Source: CAD feature listing. Evaluate the final solid. Frame: model axes, mm. Face numbers are marked on the shaded views. Give positions to 0.01 mm unless a question says otherwise; leave off trailing zeros. Loops run counter-clockwise (first coordinate to the right, second up) from the corner with the lowest first, then second, coordinate; pieces in that order, holes last.
from build123d import *

# Parameters (mm, degrees)
SALIENTE_EXTRUIR1_DEPTH = 140
SALIENTE_EXTRUIR2_START = 13.3
SALIENTE_EXTRUIR2_DEPTH = 8
SALIENTE_EXTRUIR3_START = 119
SALIENTE_EXTRUIR3_DEPTH = 8


with BuildPart() as part:
    # Croquis1 → Saliente-Extruir1 (new body)
    with BuildSketch(Plane(origin=(0, 0, 0), x_dir=(0, 0, -1), z_dir=(1, 0, 0))):
        Polygon((-70.251247354, -24.917082451), (71.151247354, 22.217082451), (70.251247354, 24.917082451), (-71.151247354, -22.217082451), align=None)
    extrude(amount=SALIENTE_EXTRUIR1_DEPTH)

    # Croquis1_3 → Saliente-Extruir2 (add)
    with BuildSketch(Plane(origin=(0, 0, 0), x_dir=(0, 0, -1), z_dir=(1, 0, 0)).offset(SALIENTE_EXTRUIR2_START)):
        Polygon((57.348752646, 17.616250882), (-39.651247354, -14.717082451), (-39.651247354, -22.717082451), (57.348752646, 9.616250882), align=None)
    extrude(amount=SALIENTE_EXTRUIR2_DEPTH)

    # Croquis1_4 → Saliente-Extruir3 (add)
    with BuildSketch(Plane(origin=(0, 0, 0), x_dir=(0, 0, -1), z_dir=(1, 0, 0)).offset(SALIENTE_EXTRUIR3_START)):
        Polygon((57.348752646, 17.616250882), (-39.651247354, -14.717082451), (-39.651247354, -22.717082451), (57.348752646, 9.616250882), align=None)
    extrude(amount=SALIENTE_EXTRUIR3_DEPTH)


solid = part.part
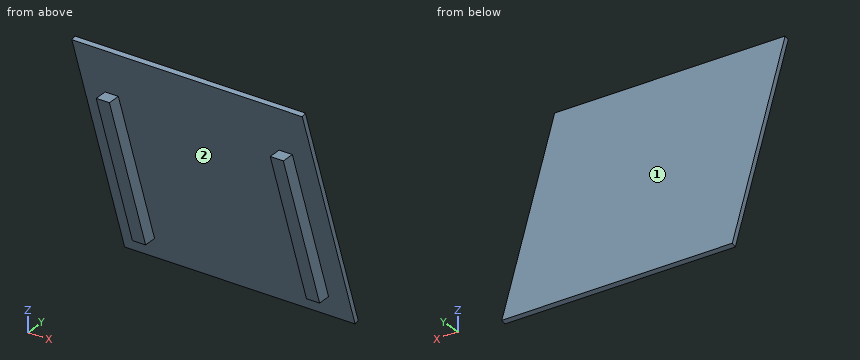
1) Contact query for flat-ended pins moving along their axis: P1, Ø20, axis at y = -7, z = -15.5, coming from the -X side; P2, Ø9, axis at x = 122.5, y = -20, coming from the +Z side; P3, Ø4, axis at x = 16.5, y = 12, coming from the -Z side; P4, Ø20, axis at y = -12, z = -20.5, coming from the +X side. Output: stop coordinate, or through.
Checks:
P1: stops at x = 13.3
P2: stops at z = 71.15
P3: stops at z = -57.35
P4: stops at x = 127
2) Pull-direction query (X, two-part tool) for the marked faces 1 and 2; classes: released by +X, released by -X, zero draft, split by the parting line, or undercut.
Checks:
face 1: zero draft
face 2: undercut
3) Cut plane D-D (x = 38.5). Return loops of the section in (y, z).
Checks:
outline: (-24.92, 70.25) - (22.22, -71.15) - (24.92, -70.25) - (-22.22, 71.15) - close
4) Ray query, probe 1 along X at (y, z) = (-17, 28); probe 2 along Y at (x, z) = (6, -40); probe 3 along Y at (x, z) = (12, 13.5). Return the intervals inside material, ascending.
Checks:
probe 1: x = 13.3 to 21.3, 119 to 127
probe 2: y = 11.83 to 14.83
probe 3: y = -6 to -3
5) Cut plane B-B (y = 14.5). Return loops of the section in (x, z).
Checks:
outline: (0, -48) - (13.3, -48) - (13.3, -57.35) - (21.3, -57.35) - (21.3, -48) - (119, -48) - (119, -57.35) - (127, -57.35) - (127, -48) - (140, -48) - (140, -39) - (0, -39) - close
6) Cut plane A-A (y = -18). Return loops of the section in (x, z).
Checks:
outline: (0, 49.5) - (140, 49.5) - (140, 58.5) - (0, 58.5) - close; (13.3, 25.5) - (21.3, 25.5) - (21.3, 39.65) - (13.3, 39.65) - close; (119, 25.5) - (127, 25.5) - (127, 39.65) - (119, 39.65) - close
7) Cut plane C-C (z = 48). Return loops of the section in (x, y), and give its area (3 significant figures).
Checks:
outline: (0, -17.5) - (140, -17.5) - (140, -14.5) - (0, -14.5) - close
area: 420 mm2
